Build history of the part. All positions in model axes, mm. A direction names the side the tool comes from. Round coordinates to 2 decimals unless told otherwise and drop trailing zeros. Write each loop counter-clockwise with the first axis right and the second up, starting at its lowest first coordinate (ties: lowest second). Pieces come first, ordered by that corner, then holes. Notation, with made-up numbers: M 19,-11 L 27,-11 A20 ccw 27,8 Z; hole C 33,20.5 d4. An arc over 180 degrees is marked long. Write item = value, one per line. Start each with the question number.
Q1. Pull direction X, two halves, no side cores. Call faces 1 (the flat face through (-63.5, 4, -6)), 2 (the flat face through (1, -42.922, -38)), 3 (the cylindrical face through (-36.98, -8.2, -34.6)), 4 (the flat face through (63.5, 4, -6)): released by +X, released by -X, zero draft, split by the parting line, or undercut.
Q2. Band-saw the part on A-A on y = -5.5. Write the cut outline in (x, z).
Q3. Probe L1, parallel to Z at x = -16, y = -34; L2, parallel to Z at x = 45, y = -7; L3, parallel to Y at x = -0.5, z = -24. List the from-to ranges inside material, lowest first.
Q4. Drop flat-ended pins along their axis: P1, Ø5, axis at x = -30, y = -6, coming from the +Z side; P2, Ø1, axis at x = -21.5, y = 4.5, coming from the -Z side; P3, Ø19, axis at x = -51.5, z = -18.5, coming from the -Y side. Give the stop position or say it passes through.
Q5. Tool access for faces 5 (the flat face through (1, -3, -0.809)), 6 (the flat face through (1, -21, -48.053)): list every direction of +Z, -Z, +X, -X, +Y, -Y with a clear straight run to the whole face (end or side of a thin tool).
Q6. Band-saw the part on B-B on z = -35.5. State how many separate pieces and enclosed holes the cut face has, plus the area to 3 significant figures.
Q7. Band-saw the part on C-C on y = -29.5. Write the cut outline in (x, z), plus the area to 3 significant figures.
```python
from build123d import *

# Parameters (mm, degrees)
BOSS_EXTRUDE1_DEPTH     = 63.5
CUT_EXTRUDE1_DEPTH      = 168.419011538
CUT_EXTRUDE1_DEPTH_BACK = 168.419011538
SKETCH2_R               = 3.175


with BuildPart() as part:
    # Sketch1 → Boss-Extrude1 (new, symmetric)
    with BuildSketch(Plane(origin=(0, 0, 0), x_dir=(0, 0, -1), z_dir=(1, 0, 0))):
        with BuildLine():
            Line((0.809260665, 1.527522938), (0.809260665, -8.632477062))
            Line((0.809260665, -8.632477062), (29.003260665, -8.632477062))
            Line((29.003260665, -8.632477062), (29.003260665, -42.922477062))
            Line((29.003260665, -42.922477062), (48.053260665, -42.922477062))
            Line((48.053260665, -42.922477062), (48.053260665, 1.527522938))
            add(Edge.make_bspline(
                [(-100.790739335, 40.936245598), (-19.432334381, 44.723152192), (48.053260665, 1.527522938)],
                knots=[0, 0, 0, 1, 1, 1], degree=2))
            add(Edge.make_bspline(
                [(-100.790739335, 40.936245598), (-95.812000817, 40.506536715), (-85.404095735, 39.35609048), (-70.04704926, 36.825372047), (-55.204457945, 33.455234316), (-41.848670928, 29.540032245), (-30.135862863, 25.255462099), (-20.192126341, 20.775035432), (-12.11168478, 16.271531389), (-5.930472237, 11.904209881), (-1.681652897, 7.768063044), (0.491896357, 4.287160304), (0.81175974, 2.163002008), (0.809260665, 1.527522938)],
                knots=[0.35379081, 0.35379081, 0.35379081, 0.35379081, 0.374279703, 0.396711254, 0.417576734, 0.436654006, 0.45374439, 0.468679994, 0.481329415, 0.491630702, 0.499615789, 0.505546281, 0.508115399, 0.508115399, 0.508115399, 0.508115399], degree=3))
        make_face()
    extrude(amount=BOSS_EXTRUDE1_DEPTH, both=True)

    # Sketch2 → Cut-Extrude1 (cut, two sides: drawn at the far end of the back side and taken through both)
    with BuildSketch(Plane(origin=(0, 0, -48.053260665), x_dir=(-1, 0, 0), z_dir=(0, 0, -1)).offset(-CUT_EXTRUDE1_DEPTH_BACK)):
        with Locations(Location((-38.1, -11.172477062, 0), (0, 0, 53.130102354))):
            Circle(SKETCH2_R)
        with Locations(Location((38.1, -11.172477062, 0), (0, 0, 53.130102354))):
            Circle(SKETCH2_R)
    extrude(amount=CUT_EXTRUDE1_DEPTH + CUT_EXTRUDE1_DEPTH_BACK, mode=Mode.SUBTRACT)


solid = part.part
```
Conclusion:
q1.face_1 = released by -X
q1.face_2 = zero draft
q1.face_3 = undercut
q1.face_4 = released by +X
q2.outline = M -63.5,-48.05 L 63.5,-48.05 L 63.5,-0.81 L -63.5,-0.81 Z
q3.L1 = -48.05 to -29
q3.L2 = -48.05 to -0.81
q3.L3 = -8.63 to 15.21
q4.P1 = -0.81
q4.P2 = -44.12
q4.P3 = -8.63
q5.face_5 = +Z, +X, -X, -Y
q5.face_6 = -Z, +X, -X, +Y, -Y
q6.separate_pieces = 1
q6.enclosed_holes = 2
q6.area = 6,540 mm^2
q7.outline = M -63.5,-48.05 L 63.5,-48.05 L 63.5,-29 L -63.5,-29 Z
q7.area = 2,420 mm^2
